Design review of the part built by this model. Coordinates are the model's own, in mm. Coordinates: 2 decimals unless noted, no trailing zeros. Loops run counter-clockwise (first coordinate to the right, second up) from the corner with the lowest first, then second, coordinate; pieces in that order, holes last. Notation, with made-up numbers: M 60.25,22.25 L 107.25,22.25 A25 ccw 107.25,35.25 Z; hole C 0,18 d8. An arc over 180 degrees is marked long. Put each result on its own line as item: value. Start each with the question number.
(1) Clearance check with a flat-ended pin moving along its axis: pin 1 (4 mm diameter, centred on x = -17.5, y = -52.5, fed in from -Z). State where the tip first meets the part, or that it passes through.
(2) Take a section at A-A, the plane y = 74.93. Give the boundary of the cut face in (x, z) (3 decimals), then the cut area to 3 significant figures.
(3) For probe 1 along Y at (x, z) = (-12, 5); probe 2 along Y at (x, z) = (61.5, 1); probe 3 along X at (y, z) = (63.5, 2.5) (3 decimals), list the stretches that pass through material, from the lowest coordinate up. Write a range as [from, to].
(4) Take a section at B-B, the plane z = 1.5. Count the separate pieces of the cut face and the enclosed holes in it, then the cut area to 3 significant figures.
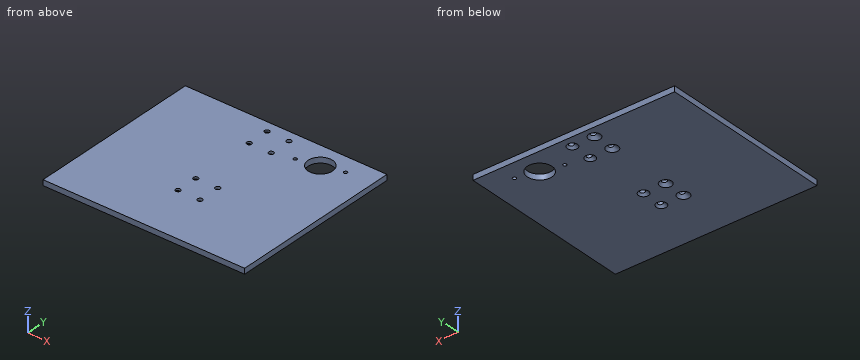
```python
from build123d import *

# Parameters (mm, degrees)
SKETCH1_W                                          = 234.95
SKETCH1_H                                          = 203.2
BOSS_EXTRUDE1_DEPTH                                = 6.35
SKETCH2_R                                          = 14.2748
CUT_EXTRUDE1_DEPTH                                 = 7.35
CSK_FOR_10_FLAT_HEAD_MACHINE_SCREW_100_D           = 5.6134
CSK_FOR_10_FLAT_HEAD_MACHINE_SCREW_100_CSINK_D     = 17.78
CSK_FOR_10_FLAT_HEAD_MACHINE_SCREW_100_CSINK_ANGLE = 90
CSK_FOR_10_FLAT_HEAD_MACHINE_SCREW_2_D             = 5.6134
CSK_FOR_10_FLAT_HEAD_MACHINE_SCREW_2_CSINK_D       = 17.78
CSK_FOR_10_FLAT_HEAD_MACHINE_SCREW_2_CSINK_ANGLE   = 90
CUT_EXTRUDE2_DEPTH                                 = 7.35


with BuildPart() as part:
    # Sketch1 → Boss-Extrude1 (new body)
    with BuildSketch(Plane.XY):
        Rectangle(SKETCH1_W, SKETCH1_H)
    extrude(amount=BOSS_EXTRUDE1_DEPTH)

    # Sketch2 → Cut-Extrude1 (cut, through all)
    with BuildSketch(Plane.XY.offset(6.35)):
        with Locations((61.595, 74.93)):
            Circle(SKETCH2_R)
    extrude(amount=-CUT_EXTRUDE1_DEPTH, mode=Mode.SUBTRACT)

    # CSK for _10 Flat Head Machine Screw _100 (through all)
    with Locations(Plane(origin=(292.076985897, -265.595089466, -43.80037576), x_dir=(0.990861087, 0, -0.134886274), z_dir=(-0.134886274, 0, -0.990861087))):
        with Locations((-308.041854919, -227.495089466), (-308.041854919, -252.895089466), (-308.041972913, -329.095089466), (-308.041972913, -354.495089466)):
            CounterSinkHole(CSK_FOR_10_FLAT_HEAD_MACHINE_SCREW_100_D / 2, CSK_FOR_10_FLAT_HEAD_MACHINE_SCREW_100_CSINK_D / 2, counter_sink_angle=CSK_FOR_10_FLAT_HEAD_MACHINE_SCREW_100_CSINK_ANGLE)

    # CSK for _10 Flat Head Machine Screw  2 (through all)
    with Locations(Plane(origin=(292.419597033, -265.595089466, -41.283588599), x_dir=(0.990861087, 0, -0.134886274), z_dir=(-0.134886274, 0, -0.990861087))):
        with Locations((-282.641854919, -227.495089466), (-282.641854919, -252.895089466), (-282.641972913, -329.095089466), (-282.641972913, -354.495089466)):
            CounterSinkHole(CSK_FOR_10_FLAT_HEAD_MACHINE_SCREW_2_D / 2, CSK_FOR_10_FLAT_HEAD_MACHINE_SCREW_2_CSINK_D / 2, counter_sink_angle=CSK_FOR_10_FLAT_HEAD_MACHINE_SCREW_2_CSINK_ANGLE)

    # Sketch10 → Cut-Extrude2 (cut, through all)
    with BuildSketch(Plane(origin=(0, 0, 0), x_dir=(-1, 0, 0), z_dir=(0, 0, -1))):
        with BuildLine():
            ThreePointArc((-85.905304985, 82.561948902), (-88.324015931, 81.043732073), (-86.805799102, 78.625021127))
            ThreePointArc((-86.805799102, 78.625021127), (-84.387088156, 80.143237956), (-85.905304985, 82.561948902))
        make_face()
        with BuildLine():
            ThreePointArc((-36.384200898, 71.234978873), (-38.802911844, 69.716762044), (-37.284695016, 67.298051098))
            ThreePointArc((-37.284695016, 67.298051098), (-34.86598407, 68.816267927), (-36.384200898, 71.234978873))
        make_face()
    extrude(amount=-CUT_EXTRUDE2_DEPTH, mode=Mode.SUBTRACT)


solid = part.part
```
Computed values:
1. pin 1: stops at z = 0
2. outline: M -117.475,0 L 47.32,0 L 47.32,6.35 L -117.475,6.35 Z; M 75.87,0 L 117.475,0 L 117.475,6.35 L 75.87,6.35 Z
2. area: 1,310 mm^2
3. probe 1: y = [-101.6, -40.9], [-35.3, -15.5], [-9.9, 60.7], [66.3, 86.1], [91.7, 101.6]
3. probe 2: y = [-101.6, 60.66], [89.2, 101.6]
3. probe 3: x = [-117.475, -17.289], [-8.864, 9.417], [15.964, 53.044], [70.146, 117.475]
4. separate pieces: 1
4. enclosed holes: 11
4. area: 46,500 mm^2
